```python
from build123d import *

# Parameters (mm, degrees)
BOSS_EXTRUDE6_DEPTH = 10
FILLET4_R           = 10
SKETCH13_R          = 4
CUT_EXTRUDE5_DEPTH  = 114.578166916
SKETCH14_R          = 10
BOSS_EXTRUDE7_DEPTH = 10
SKETCH15_R          = 4
CUT_EXTRUDE6_DEPTH  = 114.578166916
FILLET5_R           = 4
SKETCH16_R          = 11
CUT_EXTRUDE7_DEPTH  = 7


with BuildPart() as part:
    # Sketch12 → Boss-Extrude6 (new body)
    with BuildSketch(Plane(origin=(0, 0, 0), x_dir=(1, 0, 0), z_dir=(0, 1, 0))):
        with BuildLine():
            Line((-20, -50), (20, -50))
            ThreePointArc((20, -50), (28.786796564, -71.213203436), (50, -80))
            ThreePointArc((50, -80), (71.213203436, -71.213203436), (80, -50))
            Line((80, -50), (80, 50))
            ThreePointArc((80, 50), (71.213203436, 71.213203436), (50, 80))
            Line((50, 80), (-50, 80))
            ThreePointArc((-50, 80), (-71.213203436, 71.213203436), (-80, 50))
            Line((-80, 50), (-80, -50))
            ThreePointArc((-80, -50), (-71.213203436, -71.213203436), (-50, -80))
            ThreePointArc((-50, -80), (-28.786796564, -71.213203436), (-20, -50))
        make_face()
    extrude(amount=BOSS_EXTRUDE6_DEPTH)

    # Fillet4
    fillet4_edges = [part.edges().sort_by_distance(p)[0] for p in [
        (20, 5, 50),
        (-20, 5, 50),
    ]]
    fillet(fillet4_edges, radius=FILLET4_R)

    # Sketch13 → Cut-Extrude5 (cut, through all)
    with BuildSketch(Plane(origin=(0, 10, 0), x_dir=(1, 0, 0), z_dir=(0, 1, 0))):
        with Locations(Location((-55.5, 55.5, 0), (0, 0, 270))):
            Circle(SKETCH13_R)
        with Locations(Location((55.5, 55.5, 0), (0, 0, 270))):
            Circle(SKETCH13_R)
        with Locations(Location((-55.5, -55.5, 0), (0, 0, 270))):
            Circle(SKETCH13_R)
        with Locations(Location((55.5, -55.5, 0), (0, 0, 270))):
            Circle(SKETCH13_R)
    extrude(amount=-CUT_EXTRUDE5_DEPTH, mode=Mode.SUBTRACT)

    # Sketch14 → Boss-Extrude7 (add)
    with BuildSketch(Plane(origin=(0, 10, 0), x_dir=(1, 0, 0), z_dir=(0, 1, 0))):
        with Locations(Location((-55.5, 55.5, 0), (0, 0, 90))):
            Circle(SKETCH14_R)
        with Locations(Location((55.5, 55.5, 0), (0, 0, 90))):
            Circle(SKETCH14_R)
        with Locations(Location((-55.5, -55.5, 0), (0, 0, 90))):
            Circle(SKETCH14_R)
        with Locations(Location((55.5, -55.5, 0), (0, 0, 90))):
            Circle(SKETCH14_R)
    extrude(amount=BOSS_EXTRUDE7_DEPTH)

    # Sketch15 → Cut-Extrude6 (cut, through all)
    with BuildSketch(Plane.XZ.offset(-10)):
        with Locations(Location((-55.5, -55.5, 0), (0, 0, 90))):
            Circle(SKETCH15_R)
        with Locations(Location((-55.5, 55.5, 0), (0, 0, 90))):
            Circle(SKETCH15_R)
        with Locations(Location((55.5, 55.5, 0), (0, 0, 90))):
            Circle(SKETCH15_R)
        with Locations(Location((55.5, -55.5, 0), (0, 0, 90))):
            Circle(SKETCH15_R)
    extrude(amount=-CUT_EXTRUDE6_DEPTH, mode=Mode.SUBTRACT)

    # Fillet5
    fillet5_edges = [part.edges().sort_by_distance(p)[0] for p in [
        (-55.5, 10, -45.5),
        (-55.5, 10, 65.5),
        (55.5, 10, 65.5),
        (55.5, 10, -45.5),
    ]]
    fillet(fillet5_edges, radius=FILLET5_R)

    # Sketch16 → Cut-Extrude7 (cut)
    with BuildSketch(Plane(origin=(0, 10, 0), x_dir=(1, 0, 0), z_dir=(0, 1, 0))):
        with Locations(Location((0, 0, 0), (0, 0, 270))):
            Circle(SKETCH16_R)
    extrude(amount=-CUT_EXTRUDE7_DEPTH, mode=Mode.SUBTRACT)


solid = part.part
```
Geometry: final body of the model. Coordinates: model frame, mm. A direction names the side the tool comes from. Give positions to 0.01 mm unless a question says otherwise; leave off trailing zeros. Loops run counter-clockwise (first coordinate to the right, second up) from the corner with the lowest first, then second, coordinate; pieces in that order, holes last. Notation, with made-up numbers: (25, 43) -> (57, 43) arc R11 ccw to (57, 50) -> close; hole circle Ø1 at (11.5, 42). An arc over 180 degrees is marked (long way). Return JSON: item names as keys, results as strings.
Item 1: Line query: line 1 (X direction, y = 15, z = -55.5); line 2 (X direction, y = 5.25, z = 0); line 3 (Z direction, x = -55.5, y = 6.5). Output: solid intervals per line, ascending.
Filled in:
{"line 1": "-65.5 to -59.5, -51.5 to -45.5, 45.5 to 51.5, 59.5 to 65.5", "line 2": "-80 to -11, 11 to 80", "line 3": "-79.49 to -59.5, -51.5 to 51.5, 59.5 to 79.49"}
Item 2: Mould query, pull axis Z, two halves, no side actions, for faces 1 (the cylindrical face through (-70.979, 4.93, -71.445)), 2 (the cylindrical face through (-51.951, 9.86, -53.654)), 3 (the cylindrical face through (61.58, 16.96, 63.44)), 4 (the flat face through (60, 20, 56)). Classes: released by +Z, released by -Z, zero draft, split by the parting line, or undercut.
Filled in:
{"face 1": "released by -Z", "face 2": "undercut", "face 3": "undercut", "face 4": "zero draft"}
Item 3: Section A-A, the plane y = 5.5. Output: boundary loops of the cut face in (x, z).
Filled in:
{"outline": "(-80, -50) arc R30 ccw to (-50, -80) -> (50, -80) arc R30 ccw to (80, -50) -> (80, 50) arc R30 ccw to (20.95, 57.5) arc R10 cw to (11.27, 50) -> (-11.27, 50) arc R10 cw to (-20.95, 57.5) arc R30 ccw to (-80, 50) -> close; hole circle Ø8 at (-55.5, -55.5); hole circle Ø8 at (-55.5, 55.5); hole circle Ø22 at (0, 0); hole circle Ø8 at (55.5, -55.5); hole circle Ø8 at (55.5, 55.5)"}
Item 4: Section D-D, the plane z = -55.5. Output: boundary loops of the cut face in (x, y).
Filled in:
{"outline": "(-79.49, 0) -> (-59.5, 0) -> (-59.5, 20) -> (-65.5, 20) -> (-65.5, 14) arc R4 cw to (-69.5, 10) -> (-79.49, 10) -> close; (-51.5, 0) -> (51.5, 0) -> (51.5, 20) -> (45.5, 20) -> (45.5, 14) arc R4 cw to (41.5, 10) -> (-41.5, 10) arc R4 cw to (-45.5, 14) -> (-45.5, 20) -> (-51.5, 20) -> close; (59.5, 0) -> (79.49, 0) -> (79.49, 10) -> (69.5, 10) arc R4 cw to (65.5, 14) -> (65.5, 20) -> (59.5, 20) -> close"}
Item 5: Access query for faces 5 (the flat face through (-80, 5, -1)), 6 (the flat face through (0, 3, 0)), 7 (the cylindrical face through (17.32, 5.07, 52.04)). Directions: +Z, -Z, +X, -X, +Y, -Y. A direction counts if a zero-diameter tool reaches every point of the face in a straight line with its end or side. Return the directions, or none.
Filled in:
{"face 5": "+Z, -Z, -X, +Y, -Y", "face 6": "+Y", "face 7": "+Z, +Y, -Y"}
Item 6: Pin query (flat end, axial travel): P1, Ø10, axis at x = 51.5, z = 5, coming from the +Y side; P2, Ø1, axis at y = 12.5, z = 54, coming from the +X side; P3, Ø8, axis at x = -5, y = 2.5, coming from the +Z side; P4, Ø12, axis at x = -12, y = 12.5, coming from the -Z side. Return the tip coordinate at first contact, or that it passes through.
Filled in:
{"P1": "y = 10", "P2": "x = 65.94", "P3": "z = 50", "P4": "z = -80"}
Item 7: Section B-B, the plane x = 0. Output: boundary loops of the cut face in (y, z), plus the area to 3 significant figures.
Filled in:
{"outline": "(0, -80) -> (10, -80) -> (10, -11) -> (3, -11) -> (3, 11) -> (10, 11) -> (10, 50) -> (0, 50) -> close", "area": "1,150 mm^2"}
Item 8: Section C-C, the plane z = 0. Output: boundary loops of the cut face in (x, y), plus the area to 3 significant figures.
Filled in:
{"outline": "(-80, 0) -> (80, 0) -> (80, 10) -> (11, 10) -> (11, 3) -> (-11, 3) -> (-11, 10) -> (-80, 10) -> close", "area": "1,450 mm^2"}
